```python
from build123d import *

# Parameters (mm, degrees)
SKETCH1_W           = 60
SKETCH1_H           = 80
SKETCH1_R           = 1.5
SKETCH1_R_2         = 4.25
BOSS_EXTRUDE1_DEPTH = 5
SKETCH2_R           = 11
CUT_EXTRUDE1_DEPTH  = 3


with BuildPart() as part:
    # Sketch1 → Boss-Extrude1 (new body)
    with BuildSketch(Plane(origin=(0, 0, 0), x_dir=(1, 0, 0), z_dir=(0, 1, 0))):
        Rectangle(SKETCH1_W, SKETCH1_H)
        with Locations(Location((-25, 30, 0), (0, 0, 270))):
            Circle(SKETCH1_R, mode=Mode.SUBTRACT)
        with Locations(Location((25, 30, 0), (0, 0, 270))):
            Circle(SKETCH1_R, mode=Mode.SUBTRACT)
        with Locations(Location((25, 10, 0), (0, 0, 270))):
            Circle(SKETCH1_R, mode=Mode.SUBTRACT)
        with Locations(Location((25, -10, 0), (0, 0, 270))):
            Circle(SKETCH1_R, mode=Mode.SUBTRACT)
        with Locations(Location((25, -30, 0), (0, 0, 270))):
            Circle(SKETCH1_R, mode=Mode.SUBTRACT)
        with Locations(Location((-25, 10, 0), (0, 0, 270))):
            Circle(SKETCH1_R, mode=Mode.SUBTRACT)
        with Locations(Location((-25, -10, 0), (0, 0, 270))):
            Circle(SKETCH1_R, mode=Mode.SUBTRACT)
        with Locations(Location((-25, -30, 0), (0, 0, 270))):
            Circle(SKETCH1_R, mode=Mode.SUBTRACT)
        with Locations(Location((0, 0, 0), (0, 0, 270))):
            Circle(SKETCH1_R_2, mode=Mode.SUBTRACT)
    extrude(amount=BOSS_EXTRUDE1_DEPTH)

    # Sketch2 → Cut-Extrude1 (cut)
    with BuildSketch(Plane(origin=(0, 5, 0), x_dir=(1, 0, 0), z_dir=(0, 1, 0))):
        with Locations(Location((0, 0, 0), (0, 0, 270))):
            Circle(SKETCH2_R)
    extrude(amount=-CUT_EXTRUDE1_DEPTH, mode=Mode.SUBTRACT)


solid = part.part
```
The model under review builds one solid part; all positions refer to its coordinate system, in mm. A direction names the side the tool comes from. Round coordinates to 2 decimals unless told otherwise and drop trailing zeros. Loops run counter-clockwise (first coordinate to the right, second up) from the corner with the lowest first, then second, coordinate; pieces in that order, holes last.
Item 1: Mouldability with a two-part tool opening along X and no side actions: class faces 3 (the face through (-7, 5, -9)), 4 (the face through (-23.99, 2.46, 28.89)), 5 (the face through (-30, 2, 1)), 6 (the face through (-10.74, 3.52, -2.38)) as released by +X, released by -X, zero draft, split by the parting line, or undercut.
Determined:
face 3: zero draft
face 4: undercut
face 5: released by -X
face 6: undercut
Item 2: Clearance check with a flat-ended pin moving along its axis: pin 1 Ø10 at (x, z) = (0, 0) entering from +Y. State where the tip first meets the part, or that it passes through.
Determined:
pin 1: stops at y = 2
Item 3: Take a section at B-B (z = 30). Write out the cut boundary in (x, y).
Determined:
outline: (-30, 0) - (-26.5, 0) - (-26.5, 5) - (-30, 5) - close; (-23.5, 0) - (23.5, 0) - (23.5, 5) - (-23.5, 5) - close; (26.5, 0) - (30, 0) - (30, 5) - (26.5, 5) - close
Item 4: Take a section at C-C (y = 1.2). Give the number of separate pieces and of enclosed holes in the cut face, then the cut area to 3 significant figures.
Determined:
separate pieces: 1
enclosed holes: 9
area: 4,690 mm2
Item 5: For line 1 (X direction, y = 2.8, z = -30); line 2 (X direction, y = 2.3, z = 31); line 3 (X direction, y = 3.85, z = 10), list the stretches that pass through material, from the lowest coordinate up.
Determined:
line 1: x = -30 to -26.5, -23.5 to 23.5, 26.5 to 30
line 2: x = -30 to -26.12, -23.88 to 23.88, 26.12 to 30
line 3: x = -30 to -26.5, -23.5 to -4.58, 4.58 to 23.5, 26.5 to 30
Item 6: Take a section at A-A (x = 0). Write out the cut boundary in (y, z).
Determined:
outline: (0, -40) - (5, -40) - (5, -11) - (2, -11) - (2, -4.25) - (0, -4.25) - close; (0, 4.25) - (2, 4.25) - (2, 11) - (5, 11) - (5, 40) - (0, 40) - close
Item 7: For faces 1 (the face through (30, 2, 1)), 2 (the face through (-5, 2, 0)), list the 3-axis set-ups (+Z, -Z, +X, -X, +Y, -Y) from which the entire face can be reached by the end or side of a thin tool; tool diameter is ignored.
Determined:
face 1: +Z, -Z, +X, +Y, -Y
face 2: +Y
Item 8: Take a section at D-D (x = -25). Write out the cut boundary in (y, z).
Determined:
outline: (0, -40) - (5, -40) - (5, -31.5) - (0, -31.5) - close; (0, -28.5) - (5, -28.5) - (5, -11.5) - (0, -11.5) - close; (0, -8.5) - (5, -8.5) - (5, 8.5) - (0, 8.5) - close; (0, 11.5) - (5, 11.5) - (5, 28.5) - (0, 28.5) - close; (0, 31.5) - (5, 31.5) - (5, 40) - (0, 40) - close
